The model under review builds one solid part; all positions refer to its coordinate system, in mm. Coordinates: 2 decimals unless noted, no trailing zeros.
1) For line 1 (Z direction, x = -133, y = -1.8); line 2 (Z direction, x = 92.5, y = -0.6); line 3 (Z direction, x = 0, y = -2.05), list the stretches that pass through material, from the lowest coordinate up.
2) For P1, Ø6.5, axis at x = -133, z = 165, coming from the +Y side; P2, Ø9, axis at x = 140, z = -210, coming from the -Y side, all flat-tipped, find the tip position at first contact; note any pin that passes through.
3) Mouldability with a two-part tool opening along Z and no side actions: class faces 1 (the flat face through (-3, -4, 3)), 2 (the cylindrical face through (140.651, -1.972, -205.043)) as released by +Z, released by -Z, zero draft, split by the parting line, or undercut.
4) Add section A-A, the plane z = -126. Give the number of separate pieces and of enclosed holes in the cut face, then the cut area to 3 significant figures.
from build123d import *

# Parameters (mm, degrees)
F0_W     = 400
F0_H     = 450
F0_R     = 2
F1_DEPTH = 4
F2_R     = 5
F3_DEPTH = 25
F5_DEPTH = 25


with BuildPart() as f1:
    # F0 (on Front) → F1 (new body)
    with BuildSketch(Plane.XZ):
        Rectangle(F0_W, F0_H)
        with Locations((-190, 165)):
            Circle(F0_R, mode=Mode.SUBTRACT)
        with Locations((-133, 165)):
            Circle(F0_R, mode=Mode.SUBTRACT)
        with Locations((-83, 165)):
            Circle(F0_R, mode=Mode.SUBTRACT)
        with Locations((-26, 165)):
            Circle(F0_R, mode=Mode.SUBTRACT)
        with Locations((26, 165)):
            Circle(F0_R, mode=Mode.SUBTRACT)
        with Locations((83, 165)):
            Circle(F0_R, mode=Mode.SUBTRACT)
        with Locations((133, 165)):
            Circle(F0_R, mode=Mode.SUBTRACT)
        with Locations((190, 165)):
            Circle(F0_R, mode=Mode.SUBTRACT)
    extrude(amount=F1_DEPTH)

    # F2 (on face) → F3 (cut)
    with BuildSketch(Plane(origin=(0, 0, 0), x_dir=(-1, 0, 0), z_dir=(0, 1, 0))):
        with Locations((0, -210)):
            Circle(F2_R)
        with Locations((140, -210)):
            Circle(F2_R)
        with Locations((-140, -210)):
            Circle(F2_R)
    extrude(amount=-F3_DEPTH, mode=Mode.SUBTRACT)

    # F4 (on face) → F5 (cut)
    with BuildSketch(Plane(origin=(0, 0, 0), x_dir=(-1, 0, 0), z_dir=(0, 1, 0))):
        with BuildLine():
            ThreePointArc((173, -165), (175, -167), (177, -165))
            Line((177, -165), (177, -65))
            ThreePointArc((177, -65), (175, -63), (173, -65))
            Line((173, -65), (173, -165))
        make_face()
        with BuildLine():
            Line((173, 94), (173, -6))
            ThreePointArc((173, -6), (175, -8), (177, -6))
            Line((177, -6), (177, 94))
            ThreePointArc((177, 94), (175, 96), (173, 94))
        make_face()
        with BuildLine():
            Line((135, -65), (135, -165))
            ThreePointArc((135, -165), (137, -167), (139, -165))
            Line((139, -165), (139, -65))
            ThreePointArc((139, -65), (137, -63), (135, -65))
        make_face()
        with BuildLine():
            Line((135, 94), (135, -6))
            ThreePointArc((135, -6), (137, -8), (139, -6))
            Line((139, -6), (139, 94))
            ThreePointArc((139, 94), (137, 96), (135, 94))
        make_face()
        with BuildLine():
            Line((97, -65), (97, -165))
            ThreePointArc((97, -165), (99, -167), (101, -165))
            Line((101, -165), (101, -65))
            ThreePointArc((101, -65), (99, -63), (97, -65))
        make_face()
        with BuildLine():
            Line((97, 94), (97, -6))
            ThreePointArc((97, -6), (99, -8), (101, -6))
            Line((101, -6), (101, 94))
            ThreePointArc((101, 94), (99, 96), (97, 94))
        make_face()
        with BuildLine():
            Line((59, -65), (59, -165))
            ThreePointArc((59, -165), (61, -167), (63, -165))
            Line((63, -165), (63, -65))
            ThreePointArc((63, -65), (61, -63), (59, -65))
        make_face()
        with BuildLine():
            Line((59, 94), (59, -6))
            ThreePointArc((59, -6), (61, -8), (63, -6))
            Line((63, -6), (63, 94))
            ThreePointArc((63, 94), (61, 96), (59, 94))
        make_face()
        with BuildLine():
            Line((21, -65), (21, -165))
            ThreePointArc((21, -165), (23, -167), (25, -165))
            Line((25, -165), (25, -65))
            ThreePointArc((25, -65), (23, -63), (21, -65))
        make_face()
        with BuildLine():
            Line((21, 94), (21, -6))
            ThreePointArc((21, -6), (23, -8), (25, -6))
            Line((25, -6), (25, 94))
            ThreePointArc((25, 94), (23, 96), (21, 94))
        make_face()
        with BuildLine():
            Line((-17, -65), (-17, -165))
            ThreePointArc((-17, -165), (-15, -167), (-13, -165))
            Line((-13, -165), (-13, -65))
            ThreePointArc((-13, -65), (-15, -63), (-17, -65))
        make_face()
        with BuildLine():
            Line((-17, 94), (-17, -6))
            ThreePointArc((-17, -6), (-15, -8), (-13, -6))
            Line((-13, -6), (-13, 94))
            ThreePointArc((-13, 94), (-15, 96), (-17, 94))
        make_face()
        with BuildLine():
            Line((-55, -65), (-55, -165))
            ThreePointArc((-55, -165), (-53, -167), (-51, -165))
            Line((-51, -165), (-51, -65))
            ThreePointArc((-51, -65), (-53, -63), (-55, -65))
        make_face()
        with BuildLine():
            Line((-55, 94), (-55, -6))
            ThreePointArc((-55, -6), (-53, -8), (-51, -6))
            Line((-51, -6), (-51, 94))
            ThreePointArc((-51, 94), (-53, 96), (-55, 94))
        make_face()
        with BuildLine():
            Line((-93, -65), (-93, -165))
            ThreePointArc((-93, -165), (-91, -167), (-89, -165))
            Line((-89, -165), (-89, -65))
            ThreePointArc((-89, -65), (-91, -63), (-93, -65))
        make_face()
        with BuildLine():
            Line((-93, 94), (-93, -6))
            ThreePointArc((-93, -6), (-91, -8), (-89, -6))
            Line((-89, -6), (-89, 94))
            ThreePointArc((-89, 94), (-91, 96), (-93, 94))
        make_face()
        with BuildLine():
            Line((-131, -65), (-131, -165))
            ThreePointArc((-131, -165), (-129, -167), (-127, -165))
            Line((-127, -165), (-127, -65))
            ThreePointArc((-127, -65), (-129, -63), (-131, -65))
        make_face()
        with BuildLine():
            Line((-131, 94), (-131, -6))
            ThreePointArc((-131, -6), (-129, -8), (-127, -6))
            Line((-127, -6), (-127, 94))
            ThreePointArc((-127, 94), (-129, 96), (-131, 94))
        make_face()
        with BuildLine():
            Line((-169, -65), (-169, -165))
            ThreePointArc((-169, -165), (-167, -167), (-165, -165))
            Line((-165, -165), (-165, -65))
            ThreePointArc((-165, -65), (-167, -63), (-169, -65))
        make_face()
        with BuildLine():
            Line((-169, 94), (-169, -6))
            ThreePointArc((-169, -6), (-167, -8), (-165, -6))
            Line((-165, -6), (-165, 94))
            ThreePointArc((-165, 94), (-167, 96), (-169, 94))
        make_face()
    extrude(amount=-F5_DEPTH, mode=Mode.SUBTRACT)


solid = f1.part
Geometry results:
1. line 1: z = -225 to 163, 167 to 225
1. line 2: z = -225 to -166.32, -63.68 to -7.32, 95.32 to 225
1. line 3: z = -225 to -215, -205 to 225
2. P1: stops at y = 0
2. P2: passes through
3. face 1: zero draft
3. face 2: undercut
4. separate pieces: 11
4. enclosed holes: 0
4. area: 1,440 mm2
